Autodesk Inventor part; units mm, degrees
ref_plane "Work Plane1" through (-11.8427, 0, 0) normal (0, 0, -1) x (1, 0, 0)
ref_plane "YZ Plane" through (0, 0, 0) normal (1, 0, 0) x (0, 1, 0)
ref_plane "XZ Plane" through (0, 0, 0) normal (0, 1, 0) x (-1, 0, 0)
sketch "Эскиз1" plane through (0, 0, 0) normal (1, 0, 0) x (0, 1, 0)
  circle A0 centre (0, 0) radius 4
  line L0 (0, 0) -> (4, 0) construction
  line L1 (-3.9383, 0.7) -> (3.9383, 0.7)
  line L2 (-3.9383, -0.7) -> (3.9383, -0.7)
  dimension "d0" = 8
  dimension "d3" = 1.4
extrude "Базовый элемент" add sketch "Эскиз1" against normal blind 3.5
chamfer "Фаска1" distance 0.4 angle 45 1 edges at (-3.5, 3.9383, 0.7) measured on face at (-3.5, -0.0835, 1.1778)
chamfer "Фаска2" distance 0.4 angle 45 1 edges at (0, 3.9383, 0.7) measured on face at (0, 0.1896, 0.4332)
extrude "Паз" cut sketch "Эскиз1" against normal blind 1.3 contours A0 L2 L1
hole "Резьба" at (0, 0, 0) direction (-1, 0, 0) diameter 2.85 end through all
chamfer "Фаска3" distance 0.3789 angle 30 1 edges at (-3.5, 0, 1.425) measured on face at (-3.5, -2.8504, -0.1884)
ref_plane "Work Plane1" through (-11.8427, 0, 0) normal (0, 0, -1) x (1, 0, 0)
equation "\"d0\" = SD2"
equation "\"d3\" = SBR"
equation "\"d1\" = KOH"
equation "\"d8\" = PHH"
equation "\"d9\" = FAWI"
equation "\"d55\" = PHH"
equation "\"d10\" = PHH"
equation "\"d11\" = FAWI"
equation "\"d56\" = PHH"
equation "\"d4\" = STI"
equation "\"d6\" = -0.5 * GD1 + 0.5 * NND"
equation "\"d57\" = -0.5 * GD1 + 0.5 * NND"
equation "\"FAWI\" = 45deg"
equation "\"NND\" = 4"
equation "\"KOH\" = 3.5"
equation "\"SD2\" = 8"
equation "\"PHH\" = 0.4"
equation "\"SBR\" = 1.4"
equation "\"STI\" = 1.3"
equation "\"GUL\" = 0.541266 * PTC"
equation "\"THREADDIA\" = 4"
equation "\"TOA\" = 30deg"
equation "\"PTC\" = 0.7"
equation "\"GAL\" = 0.541266 * PTC"
properties part number "Гайка M4-6H ГОСТ 10657-80" material "Сталь, мягкая"
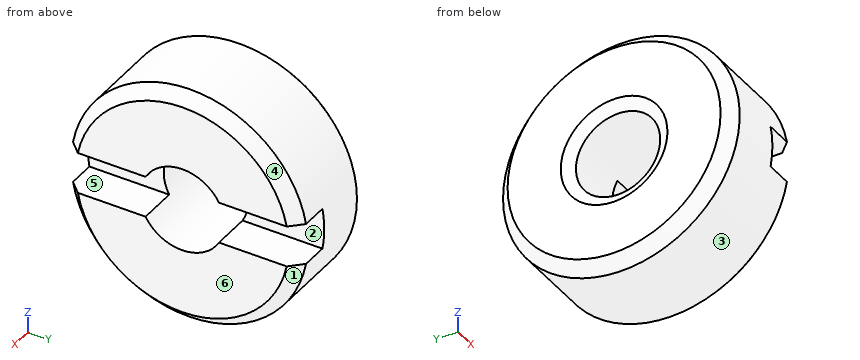
Here's how the part is built. I have some questions about the finished solid (model axes, mm). Face numbers are marked on the shaded views. A direction names the side the tool comes from. Give positions to 0.01 mm unless a question says otherwise; leave off trailing zeros. Order: outer loops, then holes, each group sorted by start corner. A loop starts at its lowest first (then second) coordinate and runs counter-clockwise, first axis right, second up. Notation, with made-up numbers: (87, 35.25) -> (110, 35.25) arc R18 cw to (110, 39.25) -> close; hole circle Ø3 at (79.25, -9). An arc over 180 degrees is marked (long way). One line per item, written item: value. Start each with the question number.
1. Imagine slicing it at B-B, the plane y = 0. List the corners of the cut face in (x, z) for me (3 decimals), plus the area to 3 significant figures.
2. Will these pins go through, and if not, where does the flat tip stop? pin 1 Ø1.5 at (x, y) = (-0.5, 1) entering from -Z; pin 2 Ø1 at (x, y) = (-1, -2) entering from -Z; pin 3 Ø1.4 at (x, y) = (-0.5, 3) entering from +Z; pin 4 Ø1.7 at (y, z) = (0, 0) entering from -X.
3. For the marked faces 1 and 2, which set-ups out of +Z, -Z, +X, -X, +Y, -Y let a thin tool reach every point of the face, with its end or its side?
4. Imagine slicing it at A-A, the plane x = -1.1. List the corners of the cut face in (y, z) for me (3 decimals), plus the area to 3 significant figures.
5. We'd pull the mould along Z, two halves only. Please class the marked faces 3, 4, 5 and 6: released by +Z, released by -Z, zero draft, split by the parting line, or undercut.
6. Imagine slicing it at C-C, the plane z = 0. List the corners of the cut face in (x, y) for me (3 decimals).
7. I need wall thicknesses on probe 1 along Z at (x, y) = (-1.9, 0) (3 decimals); probe 2 along X at (y, z) = (2.75, 0.5); probe 3 along Z at (x, y) = (-2.4, -1). Which ranges of each line are inside material? Lowest first, please. Write a range as from..to.
Values follow:
1. outline: (-3.5, -3.6) -> (-3.1, -4) -> (-0.4, -4) -> (0, -3.6) -> (0, -1.425) -> (-3.281, -1.425) -> (-3.5, -1.804) -> close; (-3.5, 1.804) -> (-3.281, 1.425) -> (0, 1.425) -> (0, 3.6) -> (-0.4, 4) -> (-3.1, 4) -> (-3.5, 3.6) -> close
1. area: 17.6 mm2
2. pin 1: stops at z = -3.99
2. pin 2: stops at z = -3.71
2. pin 3: stops at z = 3.27
2. pin 4: passes through
3. face 1: -Z, +X
3. face 2: +X, +Y, -Y
4. outline: (-3.938, -0.7) arc R4 ccw to (3.938, -0.7) -> (1.241, -0.7) arc R1.425 cw to (-1.241, -0.7) -> close; (-3.938, 0.7) -> (-1.241, 0.7) arc R1.425 cw to (1.241, 0.7) -> (3.938, 0.7) arc R4 ccw to start
4. area: 36.6 mm2
5. face 3: split by the parting line
5. face 4: released by +Z
5. face 5: undercut
5. face 6: zero draft
6. outline: (-3.5, -3.6) -> (-3.1, -4) -> (-1.3, -4) -> (-1.3, -1.425) -> (-3.281, -1.425) -> (-3.5, -1.804) -> close; (-3.5, 1.804) -> (-3.281, 1.425) -> (-1.3, 1.425) -> (-1.3, 4) -> (-3.1, 4) -> (-3.5, 3.6) -> close
7. probe 1: z = -4..-1.425, 1.425..4
7. probe 2: x = -3.5..-1.3
7. probe 3: z = -3.87..-1.02, 1.02..3.87
